```python
from build123d import *

# Parameters (mm, degrees)
SKETCH1_R                = 17.78
BOSS_EXTRUDE1_DEPTH      = 27.94
SKETCH2_R                = 11.7602
BOSS_EXTRUDE2_DEPTH      = 19.05
SKETCH3_R                = 16.637
CUT_EXTRUDE1_DEPTH       = 25.908
SKETCH4_R                = 11.049
CUT_EXTRUDE2_DEPTH       = 6.858
CUT_EXTRUDE3_DEPTH       = 38.588567411
CUT_EXTRUDE3_DEPTH_BACK  = 38.588567411
SKETCH5_W                = 5.0546
SKETCH5_H                = 12.7
BOSS_EXTRUDE3_DEPTH      = 0.9525
BOSS_EXTRUDE3_DEPTH_BACK = 0.9525
CUT_EXTRUDE4_DEPTH       = 12.192
FILLET1_R                = 2.54
CUT_EXTRUDE5_DEPTH       = 38.588567411
CUT_EXTRUDE6_REACH       = 55.295
SKETCH12_R               = 2.54


with BuildPart() as part:
    # Sketch1 → Boss-Extrude1 (new body)
    with BuildSketch(Plane(origin=(0, 0, 0), x_dir=(1, 0, 0), z_dir=(0, 1, 0))):
        with Locations(Location((0, 0, 0), (0, 0, 270))):
            Circle(SKETCH1_R)
    extrude(amount=BOSS_EXTRUDE1_DEPTH)

    # Sketch2 → Boss-Extrude2 (add)
    with BuildSketch(Plane(origin=(0, 0, 0), x_dir=(1, 0, 0), z_dir=(0, 1, 0))):
        with Locations(Location((0, 0, 0), (0, 0, 270))):
            Circle(SKETCH2_R)
    extrude(amount=-BOSS_EXTRUDE2_DEPTH)

    # Sketch3 → Cut-Extrude1 (cut)
    with BuildSketch(Plane(origin=(0, 27.94, 0), x_dir=(1, 0, 0), z_dir=(0, 1, 0))):
        with Locations(Location((0, 0, 0), (0, 0, 270))):
            Circle(SKETCH3_R)
    extrude(amount=-CUT_EXTRUDE1_DEPTH, mode=Mode.SUBTRACT)

    # Sketch4 → Cut-Extrude2 (cut)
    with BuildSketch(Plane(origin=(0, 2.032, 0), x_dir=(1, 0, 0), z_dir=(0, 1, 0))):
        with Locations(Location((0, 0, 0), (0, 0, 270))):
            Circle(SKETCH4_R)
    extrude(amount=-CUT_EXTRUDE2_DEPTH, mode=Mode.SUBTRACT)

    # Sketch5 → Cut-Extrude3 (cut, two sides: drawn at the far end of the back side and taken through both)
    with BuildSketch(Plane(origin=(0, 0, 0), x_dir=(0, 0, -1), z_dir=(1, 0, 0)).offset(-CUT_EXTRUDE3_DEPTH_BACK)):
        with Locations((9.2329, -12.7)):
            Rectangle(SKETCH5_W, SKETCH5_H)
    extrude(amount=CUT_EXTRUDE3_DEPTH + CUT_EXTRUDE3_DEPTH_BACK, mode=Mode.SUBTRACT)

    # Sketch7 → Boss-Extrude3 (add, two sides: drawn at the far end of the back side and taken through both)
    with BuildSketch(Plane(origin=(0, 0, 0), x_dir=(0, 0, -1), z_dir=(1, 0, 0)).offset(-BOSS_EXTRUDE3_DEPTH_BACK)):
        Polygon((11.7602, -6.35), (11.7602, -14.788545455), (6.7056, -19.05), (6.7056, -16.392200431), (9.7282, -13.843893442), (9.7282, -6.35), align=None)
    extrude(amount=BOSS_EXTRUDE3_DEPTH + BOSS_EXTRUDE3_DEPTH_BACK)

    # Sketch9 → Cut-Extrude4 (cut)
    with BuildSketch(Plane(origin=(0, -4.826, 0), x_dir=(1, 0, 0), z_dir=(0, 1, 0))):
        with BuildLine():
            Line((9.619493419, 5.4356), (-9.619493419, 5.4356))
            ThreePointArc((-9.619493419, 5.4356), (-2.810215135, -10.685648876), (11.049, 0))
            ThreePointArc((11.049, 0), (10.685648876, 2.810215135), (9.619493419, 5.4356))
        make_face()
    extrude(amount=-CUT_EXTRUDE4_DEPTH, mode=Mode.SUBTRACT)

    # Fillet1
    fillet1_edges = [part.edges().sort_by_distance(p)[0] for p in [
        (0, 2.032, -16.637),
    ]]
    fillet(fillet1_edges, radius=FILLET1_R)

    # Sketch11 → Cut-Extrude5 (cut, through all)
    with BuildSketch(Plane.XY):
        Polygon((-2.532708507, 7.112), (-4.7625, 7.112), (-4.7625, 12.192), (-1.27, 12.192), (-1.27, 24.638), (1.27, 24.638), (1.27, 12.192), (4.7625, 12.192), (4.7625, 7.112), (2.532708507, 7.112), align=None)
    extrude(amount=CUT_EXTRUDE5_DEPTH, mode=Mode.SUBTRACT)

    # Sketch12 → Cut-Extrude6 (cut, up to next)
    with BuildSketch(Plane.XZ.offset(19.05), mode=Mode.PRIVATE) as cut_extrude6_sk1:
        with Locations(Location((0, 0, 0), (0, 0, 270))):
            Circle(SKETCH12_R)
    cut_extrude6_tool1 = extrude(cut_extrude6_sk1.sketch, amount=-CUT_EXTRUDE6_REACH, mode=Mode.PRIVATE) & part.part
    add(cut_extrude6_tool1.solids().sort_by_distance((0, -19.05, 0))[0], mode=Mode.SUBTRACT)


solid = part.part
```
Design review of the part built by this model. Coordinates are the model's own, in mm. A direction names the side the tool comes from. Coordinates: 2 decimals unless noted, no trailing zeros. Loops run counter-clockwise (first coordinate to the right, second up) from the corner with the lowest first, then second, coordinate; pieces in that order, holes last. Notation, with made-up numbers: (7.25, 65) - (13.25, 65) arc R7 ccw to (13.25, 72) - close; hole circle Ø5 at (-31, 11.5). An arc over 180 degrees is marked (long way). Use CSV: the item, a comma, the result in double quotes. Start each with the question number.
1) For pin 1 Ø1.5 at (x, y) = (0, -11.5) entering from +Z; pin 2 Ø2 at (y, z) = (5.5, 4.5) entering from -X; pin 3 Ø2 at (x, y) = (-11, 16.5) entering from +Z, all flat-tipped, find the tip position at first contact; note any pin that passes through.
2) The part is to be moulded in two halves that separate along Z. For faces 1 (the flat face through (4.762, 9.7, 16.5)), 2 (the flat face through (-0.01, -16.89, -9.27)), 3 (the flat face through (-0.013, -15.136, -8.196)), 4 (the cylindrical face through (2.52, -18.05, 0.33)), say which applies: +Z half, -Z half, draft (parallel to the pull), parting line (faces both ways), or undercut.
3) Tool access review of faces 5 (the flat face through (-4.762, 9.6, 16.5)), 6 (the flat face through (-9.33, 2.032, 6.2)), 7 (the flat face through (-0.952, -13, -10)), 8 (the flat face through (0, -10, -9.728)): name each direction out of +Z, -Z, +X, -X, +Y, -Y from which nothing blocks a thin tool from reaching the whole face with its end or side.
4) Consider section A-A on y = -7.5. Write out the cut boundary in (x, z), then the cut area to 3 significant figures.
5) Consider section B-B on y = 15.5. Write out the cut boundary in (x, z), then the cut area to 3 significant figures.
6) Wall thickness on L1, parallel to X at y = 14, z = 0; L2, parallel to X at y = -17.7, z = 0; L3, parallel to Y at x = -8.5, z = -15: over which ranges is each line inside the solid? List them lowest first. Write a range as from..to.
Geometry says:
1,pin 1,"z = 11.76"
1,pin 2,"x = -17.43"
1,pin 3,"z = 14.7"
2,face 1,"draft"
2,face 2,"-Z half"
2,face 3,"undercut"
2,face 4,"undercut"
3,face 5,"+Z"
3,face 6,"+Y"
3,face 7,"-Z, -X, -Y"
3,face 8,"+X, -X"
4,outline,"(-9.66, -6.71) - (9.66, -6.71) arc R11.76 ccw (long way) to start; (-0.95, -11.76) - (0.95, -11.76) - (0.95, -9.73) - (-0.95, -9.73) - close; hole (-9.62, -5.44) - (9.62, -5.44) arc R11.05 ccw (long way) to start"
4,area,"63.0 mm^2"
5,outline,"(-1.27, 16.59) - (-1.27, 17.73) arc R17.78 ccw (long way) to (1.27, 17.73) - (1.27, 16.59) arc R16.64 cw (long way) to start"
5,area,"121 mm^2"
6,L1,"-17.78..-16.64, 16.64..17.78"
6,L2,"-11.76..-2.54, 2.54..11.76"
6,L3,"0..27.94"
